Input: part model. Units: mm. Frame: model coordinates. Face numbers are marked on the shaded views. A direction names the side the tool comes from. Coordinates: 2 decimals unless noted, no trailing zeros. Loops run counter-clockwise (first coordinate to the right, second up) from the corner with the lowest first, then second, coordinate; pieces in that order, holes last. Notation, with made-up numbers: M -28.75,-39.75 L 3.25,-39.75 A18 cw 3.25,-10.75 Z; hole C -10.75,-10.75 d5. An arc over 180 degrees is marked long. Use a Markdown table: item, result. Add a question column.
1. Line query: L1, parallel to Z at x = -9.5, y = 0.5; L2, parallel to X at y = 0, z = 15 (3 decimals); L3, parallel to Y at x = 13.5, z = -11.5. Output: solid intervals per line, ascending. Write a range as [from, to].
2. Section B-B on x = 0. Output: boundary loops of the cut face in (y, z), then the cut area to 3 significant figures.
3. Section C-C on z = 0. Output: boundary loops of the cut face in (x, y), then the cut area to 3 significant figures.
4. Section D-D on x = 5. Output: boundary loops of the cut face in (y, z), then the cut area to 3 significant figures.
5. Draft query along Z for the marked faces 1, 2, 3 and 4. Return one class per face: +Z half, -Z half, draft (parallel to the pull), parting line (faces both ways), or undercut.
6. Pin query (flat end, axial travel): pin 1 (3 mm diameter, centred on x = 15.5, z = -2.5, fed in from +Y); pin 2 (5 mm diameter, centred on x = -11.5, y = -3, fed in from -Z); pin 3 (1 mm diameter, centred on x = -17.5, y = 0, fed in from +Z); pin 4 (5 mm diameter, centred on x = 0, z = 0, fed in from -Y). Return the tip coordinate at first contact, or that it passes through.
7. Set-up query: the marked faces 5, 6 and 7. Return all of +Z, -Z, +X, -X, +Y, -Y with unobstructed straight access to the full face (end or side cutting, diameter ignored); none if empty.
8. Section A-A on y = -2. Output: boundary loops of the cut face in (x, z), then the cut area to 3 significant figures.
```python
from build123d import *
from build123d.topology import SkipClean

# Parameters (mm, degrees)
EXTRUDE_1_DEPTH        = 5
EXTRUDE_1_DEPTH_BACK   = 5
SKETCH_1_R             = 7.5
EXTRUDE_1_2_DEPTH      = 5
EXTRUDE_1_2_DEPTH_BACK = 5
SKETCH_1_R_2           = 24
SKETCH_1_R_3           = 20
EXTRUDE_2_DEPTH        = 3
EXTRUDE_2_DEPTH_BACK   = 3
SKETCH_1_4_R           = 20
SKETCH_1_4_R_2         = 7.5
CUT_EXTRUDE_2_DEPTH    = 6


with BuildPart() as part:
    # Sketch 1 → Extrude 1 (new, two sides: drawn at the far end of the back side and taken through both)
    with BuildSketch(Plane(origin=(0, 0, 0), x_dir=(1, 0, 0), z_dir=(0, 1, 0)).offset(-EXTRUDE_1_DEPTH_BACK)):
        with Locations(Location((0, 0, 0), (0, 0, 270))):
            Circle(SKETCH_1_R)
        with BuildLine():
            ThreePointArc((-2.132486811, -2.25), (3.1, 0), (-2.132486811, 2.25))
            Line((-2.132486811, 2.25), (-2.132486811, -2.25))
        make_face(mode=Mode.SUBTRACT)
    extrude(amount=EXTRUDE_1_DEPTH + EXTRUDE_1_DEPTH_BACK)



with BuildPart() as body_2:
    # Sketch 1 → Extrude 1 2 (new, two sides: drawn at the far end of the back side and taken through both)
    with BuildSketch(Plane(origin=(0, 0, 0), x_dir=(1, 0, 0), z_dir=(0, 1, 0)).offset(-EXTRUDE_1_2_DEPTH_BACK)):
        with Locations(Location((0, 0, 0), (0, 0, 270))):
            Circle(SKETCH_1_R_2)
        with Locations(Location((0, 0, 0), (0, 0, 270))):
            Circle(SKETCH_1_R_3, mode=Mode.SUBTRACT)
    extrude(amount=EXTRUDE_1_2_DEPTH + EXTRUDE_1_2_DEPTH_BACK)


with BuildPart() as part_1:
    add(part.part)

    add(body_2.part)  # Extrude 2 merges body 2
    # Sketch 1_4 → Extrude 2 (add, two sides: drawn at the far end of the back side and taken through both)
    with BuildSketch(Plane(origin=(0, 0, 0), x_dir=(1, 0, 0), z_dir=(0, 1, 0)).offset(-EXTRUDE_2_DEPTH_BACK)):
        with Locations(Location((0, 0, 0), (0, 0, 270))):
            Circle(SKETCH_1_4_R)
        with Locations(Location((0, 0, 0), (0, 0, 270))):
            Circle(SKETCH_1_4_R_2, mode=Mode.SUBTRACT)
    extrude(amount=EXTRUDE_2_DEPTH + EXTRUDE_2_DEPTH_BACK)

    # Sketch 3 → Cut-Extrude 2 (cut)
    with SkipClean():  # the faces are left unmerged after this step: merging them gives an invalid solid
        with BuildSketch(Plane(origin=(0, 3, 0), x_dir=(1, 0, 0), z_dir=(0, 1, 0))):
            with BuildLine():
                Line((3.847621718, 14.359519738), (1.941142838, 7.244443697))
                ThreePointArc((1.941142838, 7.244443697), (5.303300859, 5.303300859), (7.244443697, 1.941142838))
                Line((7.244443697, 1.941142838), (14.359519738, 3.847621718))
                ThreePointArc((14.359519738, 3.847621718), (15.636877848, 4.897436726), (15.687465868, 6.55006982))
                ThreePointArc((15.687465868, 6.55006982), (12.02081528, 12.02081528), (6.55006982, 15.687465868))
                ThreePointArc((6.55006982, 15.687465868), (4.897436726, 15.636877848), (3.847621718, 14.359519738))
            make_face()
            with BuildLine():
                ThreePointArc((7.244443697, -1.941142838), (5.303300859, -5.303300859), (1.941142838, -7.244443697))
                Line((1.941142838, -7.244443697), (3.847621718, -14.359519738))
                ThreePointArc((3.847621718, -14.359519738), (4.897436726, -15.636877848), (6.55006982, -15.687465868))
                ThreePointArc((6.55006982, -15.687465868), (12.02081528, -12.02081528), (15.687465868, -6.55006982))
                ThreePointArc((15.687465868, -6.55006982), (15.636877848, -4.897436726), (14.359519738, -3.847621718))
                Line((14.359519738, -3.847621718), (7.244443697, -1.941142838))
            make_face()
            with BuildLine():
                ThreePointArc((-1.941142838, -7.244443697), (-5.303300859, -5.303300859), (-7.244443697, -1.941142838))
                Line((-7.244443697, -1.941142838), (-14.359519738, -3.847621718))
                ThreePointArc((-14.359519738, -3.847621718), (-15.636877848, -4.897436726), (-15.687465868, -6.55006982))
                ThreePointArc((-15.687465868, -6.55006982), (-12.02081528, -12.02081528), (-6.55006982, -15.687465868))
                ThreePointArc((-6.55006982, -15.687465868), (-4.897436726, -15.636877848), (-3.847621718, -14.359519738))
                Line((-3.847621718, -14.359519738), (-1.941142838, -7.244443697))
            make_face()
            with BuildLine():
                ThreePointArc((-7.244443697, 1.941142838), (-5.303300859, 5.303300859), (-1.941142838, 7.244443697))
                Line((-1.941142838, 7.244443697), (-3.847621718, 14.359519738))
                ThreePointArc((-3.847621718, 14.359519738), (-4.897436726, 15.636877848), (-6.55006982, 15.687465868))
                ThreePointArc((-6.55006982, 15.687465868), (-12.02081528, 12.02081528), (-15.687465868, 6.55006982))
                ThreePointArc((-15.687465868, 6.55006982), (-15.636877848, 4.897436726), (-14.359519738, 3.847621718))
                Line((-14.359519738, 3.847621718), (-7.244443697, 1.941142838))
            make_face()
        extrude(amount=-CUT_EXTRUDE_2_DEPTH, mode=Mode.SUBTRACT)


solid = part_1.part
```
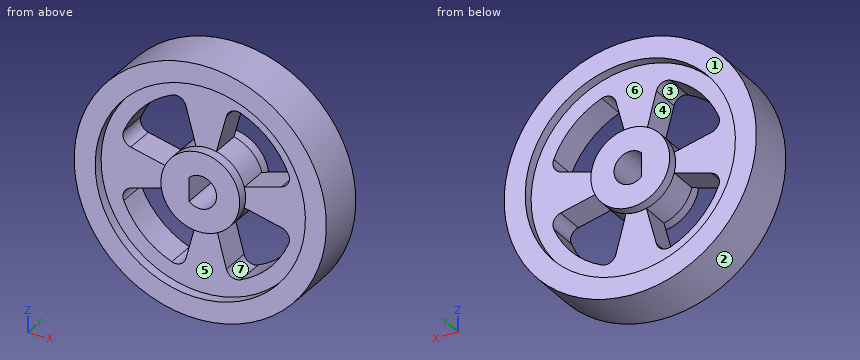
Answers below:
| question | item | result |
|---|---|---|
| 1 | L1 | z = [-22.04, -14.1], [-2.55, 2.55], [14.1, 22.04] |
| 1 | L2 | x = [-18.735, -8], [-4.149, 4.149], [8, 18.735] |
| 1 | L3 | y = [-3, 3] |
| 2 | outline | M -5,-24 L 5,-24 L 5,-20 L 3,-20 L 3,-7.5 L 5,-7.5 L 5,-3.1 L -5,-3.1 L -5,-7.5 L -3,-7.5 L -3,-20 L -5,-20 Z; M -5,3.1 L 5,3.1 L 5,7.5 L 3,7.5 L 3,20 L 5,20 L 5,24 L -5,24 L -5,20 L -3,20 L -3,7.5 L -5,7.5 Z |
| 2 | area | 318 mm² |
| 3 | outline | M -24,-5 L -20,-5 L -20,-3 L -7.5,-3 L -7.5,-5 L -2.13,-5 L -2.13,5 L -7.5,5 L -7.5,3 L -20,3 L -20,5 L -24,5 Z; M 3.1,-5 L 7.5,-5 L 7.5,-3 L 20,-3 L 20,-5 L 24,-5 L 24,5 L 20,5 L 20,3 L 7.5,3 L 7.5,5 L 3.1,5 Z |
| 3 | area | 328 mm² |
| 4 | outline | M -5,-23.47 L 5,-23.47 L 5,-19.36 L 3,-19.36 L 3,-15.68 L -3,-15.68 L -3,-19.36 L -5,-19.36 Z; M -5,-5.59 L 5,-5.59 L 5,5.59 L -5,5.59 Z; M -5,19.36 L -3,19.36 L -3,15.68 L 3,15.68 L 3,19.36 L 5,19.36 L 5,23.47 L -5,23.47 Z |
| 4 | area | 238 mm² |
| 5 | face 1 | draft |
| 5 | face 2 | parting line |
| 5 | face 3 | undercut |
| 5 | face 4 | undercut |
| 6 | pin 1 | stops at y = 3 |
| 6 | pin 2 | stops at z = -22.25 |
| 6 | pin 3 | stops at z = 16.94 |
| 6 | pin 4 | stops at y = -5 |
| 7 | face 5 | -Y |
| 7 | face 6 | +Y |
| 7 | face 7 | +Y, -Y |
| 8 | outline | C 0,0 d48; hole M -15.69,-6.55 A17 ccw -6.55,-15.69 A2 ccw -3.85,-14.36 L -1.94,-7.24 A7.5 cw -7.24,-1.94 L -14.36,-3.85 A2 ccw Z; hole M -15.69,6.55 A2 ccw -14.36,3.85 L -7.24,1.94 A7.5 cw -1.94,7.24 L -3.85,14.36 A2 ccw -6.55,15.69 A17 ccw Z; hole M -2.13,-2.25 A3.1 ccw long -2.13,2.25 Z; hole M 1.94,-7.24 L 3.85,-14.36 A2 ccw 6.55,-15.69 A17 ccw 15.69,-6.55 A2 ccw 14.36,-3.85 L 7.24,-1.94 A7.5 cw Z; hole M 1.94,7.24 A7.5 cw 7.24,1.94 L 14.36,3.85 A2 ccw 15.69,6.55 A17 ccw 6.55,15.69 A2 ccw 3.85,14.36 Z |
| 8 | area | 1,300 mm² |
